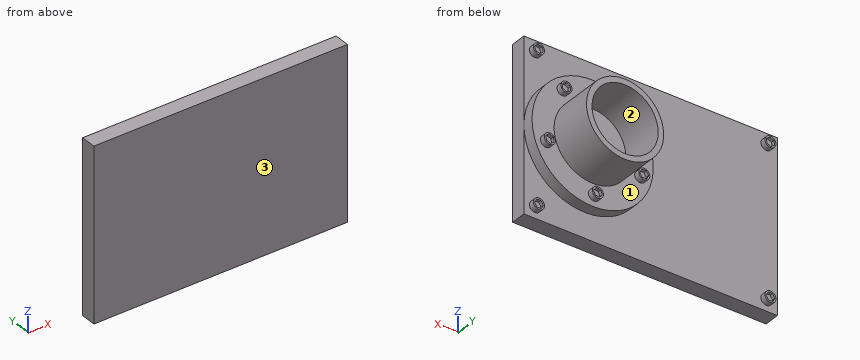
```python
from build123d import *

# Parameters (mm, degrees)
SKETCH1_W           = 230
SKETCH1_H           = 155
BOSS_EXTRUDE1_DEPTH = 14
SKETCH2_R           = 55
BOSS_EXTRUDE2_DEPTH = 10
SKETCH4_R           = 35
BOSS_EXTRUDE3_DEPTH = 40
SKETCH8_R           = 30
CUT_EXTRUDE1_DEPTH  = 40
SKETCH11_R          = 5
BOSS_EXTRUDE5_DEPTH = 5
CUT_EXTRUDE3_DEPTH  = 3
SKETCH14_R          = 5
BOSS_EXTRUDE8_DEPTH = 5
CUT_EXTRUDE4_DEPTH  = 3


with BuildPart() as part:
    # Sketch1 → Boss-Extrude1 (new body)
    with BuildSketch(Plane(origin=(0, 0, 0), x_dir=(1, 0, 0), z_dir=(0, 1, 0))):
        with Locations((115, 77.5)):
            Rectangle(SKETCH1_W, SKETCH1_H)
    extrude(amount=BOSS_EXTRUDE1_DEPTH)

    # Sketch2 → Boss-Extrude2 (add)
    with BuildSketch(Plane(origin=(0, 14, 0), x_dir=(1, 0, 0), z_dir=(0, 1, 0))):
        with Locations((175, 77.5)):
            Circle(SKETCH2_R)
    extrude(amount=BOSS_EXTRUDE2_DEPTH)

    # Sketch4 → Boss-Extrude3 (add)
    with BuildSketch(Plane(origin=(0, 24, 0), x_dir=(1, 0, 0), z_dir=(0, 1, 0))):
        with Locations(Location((175, 77.5, 0), (0, 0, 270))):
            Circle(SKETCH4_R)
    extrude(amount=BOSS_EXTRUDE3_DEPTH)

    # Sketch8 → Cut-Extrude1 (cut)
    with BuildSketch(Plane(origin=(0, 64, 0), x_dir=(1, 0, 0), z_dir=(0, 1, 0))):
        with Locations(Location((175, 77.5, 0), (0, 0, 270))):
            Circle(SKETCH8_R)
    extrude(amount=-CUT_EXTRUDE1_DEPTH, mode=Mode.SUBTRACT)

    # Sketch11 → Boss-Extrude5 (add)
    with BuildSketch(Plane(origin=(0, 14, 0), x_dir=(1, 0, 0), z_dir=(0, 1, 0))):
        with Locations(Location((10, 10, 0), (0, 0, 90))):
            Circle(SKETCH11_R)
        with Locations(Location((10, 145, 0), (0, 0, 90))):
            Circle(SKETCH11_R)
        with Locations(Location((220, 145, 0), (0, 0, 90))):
            Circle(SKETCH11_R)
        with Locations(Location((220, 10, 0), (0, 0, 90))):
            Circle(SKETCH11_R)
    extrude(amount=BOSS_EXTRUDE5_DEPTH)

    # Sketch13 → Cut-Extrude3 (cut)
    with BuildSketch(Plane(origin=(0, 19, 0), x_dir=(1, 0, 0), z_dir=(0, 1, 0))):
        Polygon((13.224457924, 12.436432727), (9.502216326, 14.010678839), (6.277758402, 11.574246112), (6.775542076, 7.563567273), (10.497783674, 5.989321161), (13.722241598, 8.425753888), align=None)
        Polygon((11.87304845, 148.581204105), (7.835110494, 148.412709592), (5.962062044, 144.831505488), (8.12695155, 141.418795895), (12.164889506, 141.587290408), (14.037937956, 145.168494512), align=None)
        Polygon((224.033447208, 145.254237993), (221.796547043, 148.620186743), (217.763099836, 148.36594875), (215.966552792, 144.745762007), (218.203452957, 141.379813257), (222.236900164, 141.63405125), align=None)
        Polygon((222.73323395, 12.977039723), (218.788424947, 13.855569896), (216.055190997, 10.878530173), (217.26676605, 7.022960277), (221.211575053, 6.144430104), (223.944809003, 9.121469827), align=None)
    extrude(amount=-CUT_EXTRUDE3_DEPTH, mode=Mode.SUBTRACT)

    # Sketch14 → Boss-Extrude8 (add)
    with BuildSketch(Plane(origin=(0, 24, 0), x_dir=(1, 0, 0), z_dir=(0, 1, 0))):
        with Locations(Location((173.870837224, 122.5, 0), (0, 0, 270))):
            Circle(SKETCH14_R)
        with Locations(Location((217.448612746, 92.479662363, 0), (0, 0, 270))):
            Circle(SKETCH14_R)
        with Locations(Location((202.363848229, 41.75794048, 0), (0, 0, 270))):
            Circle(SKETCH14_R)
        with Locations(Location((149.463175522, 40.430530026, 0), (0, 0, 270))):
            Circle(SKETCH14_R)
        with Locations(Location((131.853526279, 90.331867131, 0), (0, 0, 270))):
            Circle(SKETCH14_R)
    extrude(amount=BOSS_EXTRUDE8_DEPTH)

    # Sketch15 → Cut-Extrude4 (cut)
    with BuildSketch(Plane(origin=(0, 29, 0), x_dir=(1, 0, 0), z_dir=(0, 1, 0))):
        Polygon((221.229030496, 91.050755448), (220.576291309, 95.039146714), (216.795873559, 96.468053629), (213.668194996, 93.908569278), (214.320934183, 89.920178012), (218.101351933, 88.491271098), align=None)
        Polygon((176.398021787, 125.653834415), (172.403128782, 126.265523239), (169.875944219, 123.111688824), (171.343652661, 119.346165585), (175.338545665, 118.734476761), (177.865730228, 121.888311176), align=None)
        Polygon((202.173090327, 37.720993025), (205.764568327, 39.574265564), (205.955326229, 43.611213019), (202.554606131, 45.794887936), (198.96312813, 43.941615397), (198.772370228, 39.904667942), align=None)
        Polygon((145.564862905, 39.364466202), (148.437257567, 36.521460356), (152.335570184, 37.587524179), (153.361488139, 41.496593849), (150.489093478, 44.339599695), (146.590780861, 43.273535872), align=None)
        Polygon((129.634994486, 93.709950909), (127.818754014, 90.099604127), (130.037285808, 86.721520349), (134.072058073, 86.953783352), (135.888298544, 90.564130134), (133.669766751, 93.942213912), align=None)
    extrude(amount=-CUT_EXTRUDE4_DEPTH, mode=Mode.SUBTRACT)


solid = part.part
```
The listing builds one solid part. Answer for the finished solid, in the listing's coordinates (mm). Face numbers are marked on the shaded views. Coordinates: 2 decimals unless noted, no trailing zeros. Loops run counter-clockwise (first coordinate to the right, second up) from the corner with the lowest first, then second, coordinate; pieces in that order, holes last. Notation, with made-up numbers: M 41,-20 L 47,-20 A9 ccw 47,-4 Z; hole C -21.75,53 d8. An arc over 180 degrees is marked long. Answer as a JSON object with one key per item and string values. Group by question number.
Item 1: Section C-C (z = -66.5) is taken. Write down the section's boundary in (x, y).
Item 2: Each of these flat-tipped pins is pushed along its axis until it touches: P1, Ø5, axis at x = 150.5, z = -42.5, coming from the +Y side; P2, Ø1, axis at x = 55, z = -66.5, coming from the +Y side; P3, Ø3, axis at x = 220.5, z = -8, coming from the +Y side. Where does it stop, or does it pass through?
Item 3: Section B-B (x = 112) is taken. Write down the section's boundary in (y, z).
Item 4: Section D-D (z = -136) is taken. Write down the section's boundary in (x, y), and give its area (3 significant figures).
Item 5: Consider L1, parallel to X at y = 43, z = -77.5; L2, parallel to Y at x = 46, z = -88.5; L3, parallel to Y at x = 146, z = -83. Determine where each line is inside the solid, lowest interval first.
Item 6: Determine the mould class of the marked faces 1, 2 and 3 for opening direction Y: +Y half, -Y half, draft (parallel to the pull), parting line (faces both ways), or undercut.
Item 7: Section A-A (z = -51) is taken. Write down the section's boundary in (x, y).
Solved:
{
 "1": {"outline": "M 0,0 L 230,0 L 230,14 L 228.89,14 L 228.89,24 L 208.23,24 L 208.23,64 L 202.91,64 L 202.91,24 L 147.09,24 L 147.09,64 L 141.77,64 L 141.77,24 L 121.11,24 L 121.11,14 L 0,14 Z"},
 "2": {"P1": "stops at y = 29", "P2": "stops at y = 14", "P3": "stops at y = 16"},
 "3": {"outline": "M 0,-155 L 14,-155 L 14,0 L 0,0 Z"},
 "4": {"outline": "M 0,0 L 230,0 L 230,14 L 0,14 Z", "area": "3,220 mm2"},
 "5": {"L1": "x = 140 to 145, 205 to 210", "L2": "y = 0 to 14", "L3": "y = 0 to 24"},
 "6": {"face 1": "+Y half", "face 2": "draft", "face 3": "-Y half"},
 "7": {"outline": "M 0,0 L 230,0 L 230,14 L 223.19,14 L 223.19,24 L 197.86,24 L 197.86,64 L 189.06,64 L 189.06,24 L 160.94,24 L 160.94,64 L 152.14,64 L 152.14,24 L 126.81,24 L 126.81,14 L 0,14 Z"}
}
